Study the drawing (mm; zero at the part's minimum x, y, z) and answer. A direction names the side the tool comes from. Coordinates: 2 decimals unless noted, no trailing zeros. Order: outer loops, then holes, each group sorted by start corner. A loop starts at its lowest first (then second) coordinate and runs counter-clockwise, first axis right, second up. Notation, with made-up numbers: (5, 85.5) -> (55, 85.5) arc R24 ccw to (55, 111.5) -> close; hole circle Ø3 at (46, 13). An arc over 180 degrees is marked (long way). Write each question's results on one line, items separated by ' | '. Start each with the question number.
(1) The part is cut by section C-C, the plane z = 2.6. Give the vertices of the cut face in (x, y), then the cut area to 3 significant figures.
(2) Given pin 1 (1.5 mm diameter, centred on x = 20, y = 10.5, fed in from +Z), flat-ended and moving along its own axis, determine where the tip first touches the part or whether it passes through.
(3) Straight lines are drawn through the part: L1, parallel to Y at x = 18.8, z = 3.7; L2, parallel to X at y = 6.5, z = 1.35; L3, parallel to X at y = 2.25, z = 4.2. For each, find the intervals that lie inside material, in ascending order.
(4) Determine the mould class of the marked faces 1, 2 and 3 for opening direction X: +X half, -X half, draft (parallel to the pull), parting line (faces both ways), or undercut.
(5) The part is cut by section B-B, the plane y = 7.5. Give the vertices of the cut face in (x, z), then the cut area to 3 significant figures.
(6) The part is cut by section D-D, the plane x = 3.8. Give the vertices of the cut face in (y, z).
(7) The part is cut by section A-A, the plane x = 18.8. Give the vertices of the cut face in (y, z), then the cut area to 3 significant figures.
(8) A tool of negligible diameter and unlimited length cuts with its end or side. For the marked faces 4 and 5, from which of +Z, -Z, +X, -X, +Y, -Y can it reach the whole face along a straight path? Write none if from no direction.
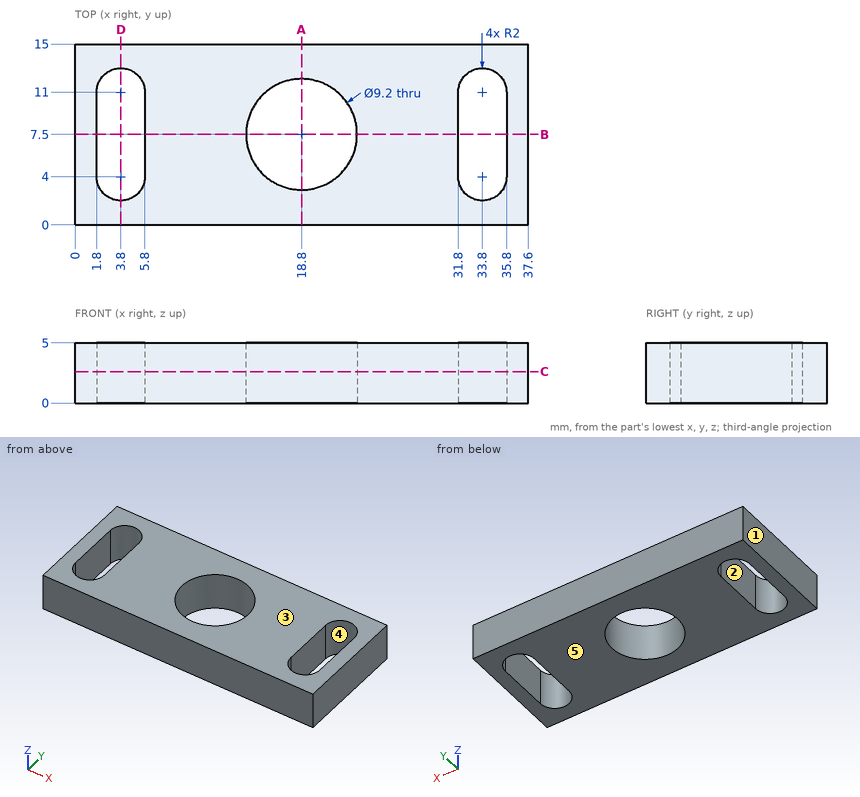
Established:
1) outline: (0, 0) -> (37.6, 0) -> (37.6, 15) -> (0, 15) -> close; hole (1.8, 4) arc R2 ccw to (5.8, 4) -> (5.8, 11) arc R2 ccw to (1.8, 11) -> close; hole circle Ø9.2 at (18.8, 7.5); hole (31.8, 4) arc R2 ccw to (35.8, 4) -> (35.8, 11) arc R2 ccw to (31.8, 11) -> close | area: 416 mm^2
2) pin 1: passes through
3) L1: y = 0 to 2.9, 12.1 to 15 | L2: x = 0 to 1.8, 5.8 to 14.31, 23.29 to 31.8, 35.8 to 37.6 | L3: x = 0 to 2.83, 4.77 to 32.83, 34.77 to 37.6
4) face 1: -X half | face 2: undercut | face 3: draft
5) outline: (0, 0) -> (1.8, 0) -> (1.8, 5) -> (0, 5) -> close; (5.8, 0) -> (14.2, 0) -> (14.2, 5) -> (5.8, 5) -> close; (23.4, 0) -> (31.8, 0) -> (31.8, 5) -> (23.4, 5) -> close; (35.8, 0) -> (37.6, 0) -> (37.6, 5) -> (35.8, 5) -> close | area: 102 mm^2
6) outline: (0, 0) -> (2, 0) -> (2, 5) -> (0, 5) -> close; (13, 0) -> (15, 0) -> (15, 5) -> (13, 5) -> close
7) outline: (0, 0) -> (2.9, 0) -> (2.9, 5) -> (0, 5) -> close; (12.1, 0) -> (15, 0) -> (15, 5) -> (12.1, 5) -> close | area: 29.0 mm^2
8) face 4: +Z, -Z | face 5: -Z, +X, -X, +Y, -Y
